Build history of the part. All positions in model axes, mm. A direction names the side the tool comes from. Give positions to 0.01 mm unless a question says otherwise; leave off trailing zeros. Write each loop counter-clockwise with the first axis right and the second up, starting at its lowest first coordinate (ties: lowest second). Pieces come first, ordered by that corner, then holes. Notation, with made-up numbers: M -31,47.25 L 13,47.25 A33 cw 13,82.25 Z; hole C 51,74 d9. An arc over 180 degrees is marked long. One line per item, written item: value. Start each with the question number.
from build123d import *

# Parameters (mm, degrees)
SKETCH3_R           = 1.7
BOSS_EXTRUDE1_DEPTH = 3.5
BOSS_EXTRUDE2_DEPTH = 2
FILLET1_R           = 2
SKETCH5_R           = 1.7
CUT_EXTRUDE1_DEPTH  = 4
FILLET2_R           = 3


with BuildPart() as part:
    # Sketch3 → Boss-Extrude1 (new body)
    with BuildSketch(Plane.XY):
        with BuildLine():
            Line((-19, -3), (19, -3))
            ThreePointArc((19, -3), (19.707106781, -2.707106781), (20, -2))
            Line((20, -2), (20, 2))
            ThreePointArc((20, 2), (19.707106781, 2.707106781), (19, 3))
            Line((19, 3), (-19, 3))
            ThreePointArc((-19, 3), (-19.707106781, 2.707106781), (-20, 2))
            Line((-20, 2), (-20, -2))
            ThreePointArc((-20, -2), (-19.707106781, -2.707106781), (-19, -3))
        make_face()
        with Locations((-16, 0)):
            Circle(SKETCH3_R, mode=Mode.SUBTRACT)
        with Locations(Location((16, 0, 0), (0, 0, 180))):
            Circle(SKETCH3_R, mode=Mode.SUBTRACT)
    extrude(amount=BOSS_EXTRUDE1_DEPTH)

    # Sketch4 → Boss-Extrude2 (add, symmetric)
    with BuildSketch(Plane(origin=(0, 0, 0), x_dir=(0, 0, -1), z_dir=(1, 0, 0))):
        Polygon((0, 3), (11.5, -22), (-3.5, -22), (-3.5, 3), align=None)
    extrude(amount=BOSS_EXTRUDE2_DEPTH, both=True)

    # Fillet1
    # the kernel refuses this fillet: 2 mm, written as the material it adds along each edge
    with BuildSketch(Plane(origin=(2, -3, 0), x_dir=(1, 0, 0), z_dir=(0, 0, 1))) as fillet1_piece_1:
        with BuildLine():
            CenterArc((FILLET1_R, -FILLET1_R), FILLET1_R, 90, 90)
            Line((0, -FILLET1_R), (0, 0))
            Line((0, 0), (FILLET1_R, 0))
        make_face()
    extrude(amount=3.5)
    with BuildSketch(Plane(origin=(-2, 3, 0), x_dir=(0, 0, -1), z_dir=(0, -1, 0))) as fillet1_piece_2_section:
        with BuildLine():
            CenterArc((FILLET1_R, -FILLET1_R), FILLET1_R, 90, 90)
            Line((0, -FILLET1_R), (0, 0))
            Line((0, 0), (FILLET1_R, 0))
        make_face()
    fillet1_piece_2 = extrude(amount=6, mode=Mode.PRIVATE)
    fillet1_piece_2 = split(fillet1_piece_2, bisect_by=Plane(origin=(-2.500058987, 0.046625327, -1.35855235), z_dir=(3.171977462044394e-15, -0.4179056082321443, 0.9084904526785746)), keep=Keep.TOP, mode=Mode.PRIVATE)
    add(fillet1_piece_2)
    with BuildSketch(Plane(origin=(2, 3, 0), x_dir=(0, 0, -1), z_dir=(0, -1, 0))) as fillet1_piece_3_section:
        with BuildLine():
            CenterArc((FILLET1_R, FILLET1_R), FILLET1_R, 180, 90)
            Line((0, FILLET1_R), (0, 0))
            Line((0, 0), (FILLET1_R, 0))
        make_face()
    fillet1_piece_3 = extrude(amount=6, mode=Mode.PRIVATE)
    fillet1_piece_3 = split(fillet1_piece_3, bisect_by=Plane(origin=(2.500058987, 0.046625327, -1.35855235), z_dir=(3.171977462044394e-15, -0.4179056082321443, 0.9084904526785746)), keep=Keep.TOP, mode=Mode.PRIVATE)
    add(fillet1_piece_3)
    with BuildSketch(Plane(origin=(-2, -3, 0), x_dir=(-1, 0, 0), z_dir=(0, 0, 1))) as fillet1_piece_4:
        with BuildLine():
            CenterArc((FILLET1_R, FILLET1_R), FILLET1_R, 180, 90)
            Line((0, FILLET1_R), (0, 0))
            Line((0, 0), (FILLET1_R, 0))
        make_face()
    extrude(amount=3.5)
    with BuildSketch(Plane(origin=(2, -3, -5), x_dir=(1, 0, 0), z_dir=(0, 0, 1))) as fillet1_piece_5a_section:
        with BuildLine():
            CenterArc((FILLET1_R, -FILLET1_R), FILLET1_R, 90, 90)
            Line((0, -FILLET1_R), (0, 0))
            Line((0, 0), (FILLET1_R, 0))
        make_face()
    fillet1_piece_5a = extrude(amount=8.5, mode=Mode.PRIVATE)
    fillet1_piece_5a = split(fillet1_piece_5a, bisect_by=Plane(origin=(2.435770174, -3.481600485, 0), z_dir=(0, 0, -1)), keep=Keep.TOP, mode=Mode.PRIVATE)
    fillet1_piece_5a = split(fillet1_piece_5a, bisect_by=Plane(origin=(2.435770174, -2.915610611, -2.721180881), z_dir=(3.171977462044394e-15, -0.4179056082321443, 0.9084904526785746)), keep=Keep.TOP, mode=Mode.PRIVATE)
    with BuildSketch(Plane(origin=(2, 3, 0), x_dir=(0, 0, -1), z_dir=(0, -1, 0))) as fillet1_piece_5b_section:
        with BuildLine():
            CenterArc((FILLET1_R, FILLET1_R), FILLET1_R, 180, 90)
            Line((0, FILLET1_R), (0, 0))
            Line((0, 0), (FILLET1_R, 0))
        make_face()
    fillet1_piece_5b = extrude(amount=11, mode=Mode.PRIVATE)
    fillet1_piece_5b = split(fillet1_piece_5b, bisect_by=Plane(origin=(2.452790229, -3, -0.452790229), z_dir=(0, -1, 0)), keep=Keep.TOP, mode=Mode.PRIVATE)
    fillet1_piece_5 = fillet1_piece_5a & fillet1_piece_5b
    add(fillet1_piece_5)
    with BuildSketch(Plane(origin=(-2, -3, -5), x_dir=(-1, 0, 0), z_dir=(0, 0, 1))) as fillet1_piece_6a_section:
        with BuildLine():
            CenterArc((FILLET1_R, FILLET1_R), FILLET1_R, 180, 90)
            Line((0, FILLET1_R), (0, 0))
            Line((0, 0), (FILLET1_R, 0))
        make_face()
    fillet1_piece_6a = extrude(amount=8.5, mode=Mode.PRIVATE)
    fillet1_piece_6a = split(fillet1_piece_6a, bisect_by=Plane(origin=(-2.435770174, -3.481600485, 0), z_dir=(0, 0, -1)), keep=Keep.TOP, mode=Mode.PRIVATE)
    fillet1_piece_6a = split(fillet1_piece_6a, bisect_by=Plane(origin=(-2.435770174, -2.915610611, -2.721180881), z_dir=(3.171977462044394e-15, -0.4179056082321443, 0.9084904526785746)), keep=Keep.TOP, mode=Mode.PRIVATE)
    with BuildSketch(Plane(origin=(-2, 3, 0), x_dir=(0, 0, -1), z_dir=(0, -1, 0))) as fillet1_piece_6b_section:
        with BuildLine():
            CenterArc((FILLET1_R, -FILLET1_R), FILLET1_R, 90, 90)
            Line((0, -FILLET1_R), (0, 0))
            Line((0, 0), (FILLET1_R, 0))
        make_face()
    fillet1_piece_6b = extrude(amount=11, mode=Mode.PRIVATE)
    fillet1_piece_6b = split(fillet1_piece_6b, bisect_by=Plane(origin=(-2.452790229, -3, -0.452790229), z_dir=(0, -1, 0)), keep=Keep.TOP, mode=Mode.PRIVATE)
    fillet1_piece_6 = fillet1_piece_6a & fillet1_piece_6b
    add(fillet1_piece_6)
    # the kernel refuses this fillet: 2 mm, written as the material it takes off along each edge
    with BuildSketch(Plane(origin=(7, -22, 3.5), x_dir=(0, 0, -1), z_dir=(-1, 0, 0))) as fillet1_2_piece_1:
        with BuildLine():
            CenterArc((FILLET1_R, -FILLET1_R), FILLET1_R, 90, 90)
            Line((0, -FILLET1_R), (0, 0))
            Line((0, 0), (FILLET1_R, 0))
        make_face()
    extrude(amount=14, mode=Mode.SUBTRACT)

    # Sketch5 → Cut-Extrude1 (cut)
    with BuildSketch(Plane(origin=(2, 0, 0), x_dir=(0, 0, -1), z_dir=(1, 0, 0))):
        with Locations((6.615815201, -18.97305612)):
            Circle(SKETCH5_R)
    extrude(amount=-CUT_EXTRUDE1_DEPTH, mode=Mode.SUBTRACT)

    # Fillet2
    fillet2_edges = [part.edges().sort_by_distance(p)[0] for p in [
        (0, -22, -11.5),
    ]]
    fillet(fillet2_edges, radius=FILLET2_R)


solid = part.part
1) Probe line 1 along Y through (x, z) = (16, 1.15); line 2 along X through (y, z) = (-13.5, -7); line 3 along Z through (x, y) = (14.5, 1). List the from-to ranges inside material, lowest first. Write a range as from..to.
2) Band-saw the part on A-A (x = -16). List the corners of the cut face in (y, z).
3) Band-saw the part on C-C (y = 0). List the corners of the cut face in (x, z), then the cut area to 3 significant figures.
4) Tool access for faces 5 (the face through (12, 0, 0)), 6 (the face through (0, 3, 2)): list every direction of +Z, -Z, +X, -X, +Y, -Y with a clear straight run to the whole face (end or side of a thin tool).
5) Band-saw the part on B-B (z = -6). List the corners of the cut face in (x, y).
6) Drop flat-ended pins along their axis: P1, Ø4, axis at y = -7.5, z = -4, coming from the +X side; P2, Ø5, axis at x = -13.5, y = -1, coming from the -Z side; P3, Ø1.5, axis at x = 13.5, z = 0, coming from the -Y side. Give the stop position or say it passes through.
7) Mould opens along X. For faces 1 (the face through (-14.43, -0.65, 1.73)), 2 (the face through (2.6, -3.57, 1.32)), 3 (the face through (14.43, 0.65, 1.73)), 4 (the face through (-2.57, -3.6, 1.32)) say: released by +X, released by -X, zero draft, split by the parting line, or undercut.
8) Band-saw the part on D-D (x = 1.5). List the corners of the cut face in (y, z).
Model answer:
1. line 1: y = -3..-1.7, 1.7..3
1. line 2: x = -2..2
1. line 3: z = 0..3.5
2. outline: M -3,0 L -1.7,0 L -1.7,3.5 L -3,3.5 Z; M 1.7,0 L 3,0 L 3,3.5 L 1.7,3.5 Z
3. outline: M -20,0 L -17.7,0 L -17.7,3.5 L -20,3.5 Z; M -14.3,0 L -4,0 A2 cw -2.1,-1.38 L 2.1,-1.38 A2 cw 4,0 L 14.3,0 L 14.3,3.5 L -14.3,3.5 Z; M 17.7,0 L 20,0 L 20,3.5 L 17.7,3.5 Z
3. area: 123 mm²
4. face 5: -Z, +X, +Y, -Y
4. face 6: +Z, -Z, +X, -X, +Y
5. outline: M -2,-22 L 2,-22 L 2,-20.56 L -2,-20.56 Z; M -2,-17.39 L 2,-17.39 L 2,-10.04 L -2,-10.04 Z
6. P1: stops at x = 2
6. P2: stops at z = 0
6. P3: stops at y = -3
7. face 1: undercut
7. face 2: released by +X
7. face 3: undercut
7. face 4: released by -X
8. outline: M -22,-6.82 A3 ccw -17.75,-9.54 L 3,0 L 3,3.5 L -20,3.5 A2 ccw -22,1.5 Z; hole C -18.97,-6.62 d3.4
